Part model, mm, in its own coordinate system. A direction names the side the tool comes from. Give positions to 0.01 mm unless a question says otherwise; leave off trailing zeros. Loops run counter-clockwise (first coordinate to the right, second up) from the corner with the lowest first, then second, coordinate; pieces in that order, holes last. Notation, with made-up numbers: M 11.25,-3 L 41.25,-3 A21 cw 41.25,4 Z; hole C -36.5,-26.5 d7. An arc over 180 degrees is marked long. Answer in a Markdown table with one row per item.
from build123d import *

# Parameters (mm, degrees)
VISTA_FRONTAL_W         = 59.3
VISTA_FRONTAL_H         = 29
VISTA_FRONTAL_W_2       = 52.3
VISTA_FRONTAL_H_2       = 24
CORPO_DO_MODULO_DEPTH   = 15.65
ESBO_O3_R               = 2.3
PADR_O_DE_ENCAIXE_DEPTH = 45.328828092
ESBO_O4_R               = 2
ESBO_O4_W               = 3
ESBO_O4_H               = 16
FUROS_INTERNOS_DEPTH    = 3.6
CAL_O_SUPERIOR_DEPTH    = 2
CORTE_START             = -0.5
FURO_COMPENSADOR_R      = 2.3
CORTE_COMPENSADOR_DEPTH = 0.5


with BuildPart() as part:
    # Vista Frontal → Corpo do Modulo (new, symmetric)
    with BuildSketch(Plane.XY):
        Rectangle(VISTA_FRONTAL_W, VISTA_FRONTAL_H)
        Rectangle(VISTA_FRONTAL_W_2, VISTA_FRONTAL_H_2, mode=Mode.SUBTRACT)
    extrude(amount=CORPO_DO_MODULO_DEPTH, both=True)

    # Esboço3 → Padrão de Encaixe (cut, through all)
    with BuildSketch(Plane(origin=(0, 14.5, 0), x_dir=(1, 0, 0), z_dir=(0, 1, 0))):
        with Locations((-29.65, 0)):
            Circle(ESBO_O3_R)
        Polygon((26.6477786, -15.65), (29.65, -10.45), (29.65, -15.65), align=None)
        Polygon((29.65, 15.65), (26.6477786, 15.65), (29.65, 10.45), align=None)
    extrude(amount=-PADR_O_DE_ENCAIXE_DEPTH, mode=Mode.SUBTRACT)

    # Esboço4 → Furos Internos (cut)
    with BuildSketch(Plane.XZ.offset(14.5)):
        with Locations(Location((0.15, 0, 0), (0, 0, 270))):
            Circle(ESBO_O4_R)
        with Locations(Location((-2.85, 9.5, 0), (0, 0, 270))):
            Circle(ESBO_O4_R)
        with Locations(Location((-12.85, 9.5, 0), (0, 0, 270))):
            Circle(ESBO_O4_R)
        with Locations(Location((-12.85, 3.5, 0), (0, 0, 270))):
            Circle(ESBO_O4_R)
        with Locations(Location((-12.85, -3.5, 0), (0, 0, 90))):
            Circle(ESBO_O4_R)
        with Locations(Location((-12.85, -9.5, 0), (0, 0, 90))):
            Circle(ESBO_O4_R)
        with Locations(Location((-2.85, -9.5, 0), (0, 0, 90))):
            Circle(ESBO_O4_R)
        with Locations((6.15, 0)):
            Rectangle(ESBO_O4_W, ESBO_O4_H)
    extrude(amount=-FUROS_INTERNOS_DEPTH, mode=Mode.SUBTRACT)

    # Extra Tampa → Calço Superior (add)
    with BuildSketch(Plane(origin=(0, 14.5, 0), x_dir=(1, 0, 0), z_dir=(0, 1, 0))):
        Polygon((-29.65, 15.65), (22.443633412, 15.65), (25.85, 10.1), (25.85, -10.1), (22.443633412, -15.65), (-29.65, -15.65), align=None)
    extrude(amount=CAL_O_SUPERIOR_DEPTH)

    # Furo Compensador → Corte compensador (cut)
    with BuildSketch(Plane.XZ.offset(-14.5).offset(CORTE_START)):
        with Locations((-29.65, 0)):
            Circle(FURO_COMPENSADOR_R)
    extrude(amount=CORTE_COMPENSADOR_DEPTH, mode=Mode.SUBTRACT)


solid = part.part
(1) Pin check, flat tip, straight feed: pin 1 Ø3.5 at (x, z) = (-12.85, -9.5) entering from -Y. Stop position of the tip, or through.
Recorded:
| item | result |
|---|---|
| pin 1 | stops at y = 12 |
(2) Saw through at C-C (x = -12.85). Write the cut outline in (y, z).
Recorded:
| item | result |
|---|---|
| outline | M -14.5,-15.65 L -12,-15.65 L -12,-11.5 L -14.5,-11.5 Z; M -14.5,-7.5 L -12,-7.5 L -12,-5.5 L -14.5,-5.5 Z; M -14.5,-1.5 L -12,-1.5 L -12,1.5 L -14.5,1.5 Z; M -14.5,5.5 L -12,5.5 L -12,7.5 L -14.5,7.5 Z; M -14.5,11.5 L -12,11.5 L -12,15.65 L -14.5,15.65 Z; M 12,-15.65 L 16.5,-15.65 L 16.5,15.65 L 12,15.65 Z |
(3) Saw through at B-B (z = 0). Write the cut outline in (x, y), plus the area to 3 significant figures.
Recorded:
| item | result |
|---|---|
| outline | M -29.65,15 L -27.35,15 L -27.35,-14.5 L -1.85,-14.5 L -1.85,-12 L -26.15,-12 L -26.15,12 L 26.15,12 L 26.15,-12 L 7.65,-12 L 7.65,-14.5 L 29.65,-14.5 L 29.65,14.5 L 25.85,14.5 L 25.85,16.5 L -29.65,16.5 Z; M 2.15,-14.5 L 4.65,-14.5 L 4.65,-12 L 2.15,-12 Z |
| area | 490 mm^2 |
(4) Pull direction X, two halves, no side cores. Call faces 1 (the face through (24.123, 15.486, -12.914)), 2 (the face through (-5.5, 12.4, 15.65)), 3 (the face through (-4.833, -13.268, -9.76)): +X half, -X half, draft (parallel to the pull), parting line (faces both ways), or undercut.
Recorded:
| item | result |
|---|---|
| face 1 | +X half |
| face 2 | draft |
| face 3 | undercut |
(5) Saw through at D-D (x = -2.85). Write the cut outline in (y, z).
Recorded:
| item | result |
|---|---|
| outline | M -14.5,-15.65 L -12,-15.65 L -12,-11.5 L -14.5,-11.5 Z; M -14.5,-7.5 L -12,-7.5 L -12,7.5 L -14.5,7.5 Z; M -14.5,11.5 L -12,11.5 L -12,15.65 L -14.5,15.65 Z; M 12,-15.65 L 16.5,-15.65 L 16.5,15.65 L 12,15.65 Z |
(6) Saw through at A-A (y = -5). Write the cut outline in (x, z), plus the area to 3 significant figures.
Recorded:
| item | result |
|---|---|
| outline | M -29.65,-15.65 L -26.15,-15.65 L -26.15,15.65 L -29.65,15.65 L -29.65,2.3 A2.3 cw -29.65,-2.3 Z; M 26.15,-15.65 L 26.65,-15.65 L 29.65,-10.45 L 29.65,10.45 L 26.65,15.65 L 26.15,15.65 Z |
| area | 195 mm^2 |
(7) Which spindle directions (+Z, -Z, +X, -X, +Y, -Y) get a long thin tool onto all of the face, cutting with end or side? Do faces 4 (the face through (-26.15, 0, 0)), 5 (the face through (6, -13, -8)), 6 (the face through (24.17, 15.49, 12.84)). Say none if no direction does.
Recorded:
| item | result |
|---|---|
| face 4 | +Z, -Z |
| face 5 | -Y |
| face 6 | +Z, +X, +Y |
(8) Drill centre lines: line 1 along Y through (x, z) = (-3, -4); line 2 along X through (y, z) = (-13, 9); line 3 along Z through (x, y) = (-12, -13). Where is each one in solid material? Low to high.
Recorded:
| item | result |
|---|---|
| line 1 | y = -14.5 to -12, 12 to 16.5 |
| line 2 | x = -29.65 to -14.79, -10.91 to -4.79, -0.91 to 29.65 |
| line 3 | z = -15.65 to -11.31, -7.69 to -5.31, -1.69 to 1.69, 5.31 to 7.69, 11.31 to 15.65 |
